Verification items for the finished model (mm, model axes). A direction names the side the tool comes from. Coordinates: 2 decimals unless noted, no trailing zeros. Write each loop counter-clockwise with the first axis right and the second up, starting at its lowest first coordinate (ties: lowest second). Pieces come first, ordered by that corner, then holes. Notation, with made-up numbers: (44, 54) -> (61, 54) arc R26 ccw to (61, 85) -> close; hole circle Ø8 at (40, -20.75). An arc over 180 degrees is marked (long way). Answer in a Markdown table with one row per item.
```python
from build123d import *

# Parameters (mm, degrees)
SKETCH_1_R          = 23.15
EXTRUDE_1_DEPTH     = 1.2
SKETCH_2_R          = 1
CUT_EXTRUDE_1_DEPTH = 1.6


with BuildPart() as part:
    # 草图1 → 凸台-拉伸1 (new body)
    with BuildSketch(Plane(origin=(0, 0, 0), x_dir=(1, 0, 0), z_dir=(0, 1, 0))):
        with Locations(Location((0, 0, 0), (0, 0, 270))):
            Circle(SKETCH_1_R)
    extrude(amount=EXTRUDE_1_DEPTH)

    # 草图2 → 切除-拉伸1 (cut)
    with BuildSketch(Plane(origin=(0, 1.2, 0), x_dir=(1, 0, 0), z_dir=(0, 1, 0))):
        with Locations(Location((0, 20.5, 0), (0, 0, 270))):
            Circle(SKETCH_2_R)
        with Locations(Location((14.495689014, 14.495689014, 0), (0, 0, 270))):
            Circle(SKETCH_2_R)
        with Locations(Location((14.495689014, -14.495689014, 0), (0, 0, 270))):
            Circle(SKETCH_2_R)
        with Locations(Location((0, -20.5, 0), (0, 0, 270))):
            Circle(SKETCH_2_R)
        with Locations(Location((-14.495689014, -14.495689014, 0), (0, 0, 270))):
            Circle(SKETCH_2_R)
        with Locations(Location((-14.495689014, 14.495689014, 0), (0, 0, 270))):
            Circle(SKETCH_2_R)
        Polygon((23.15, 0), (23.15, 4), (9.15, 4), (9.15, -4), (23.15, -4), align=None)
    extrude(amount=-CUT_EXTRUDE_1_DEPTH, mode=Mode.SUBTRACT)


solid = part.part
```
1. Mould release check, pull along Z, two halves, no side actions. Record for faces 3 (the cylindrical face through (-15.472, 0.608, 14.279)), 4 (the cylindrical face through (-23.13, 0.59, -0.96)), 5 (the flat face through (0, 1.2, 0)): released by +Z, released by -Z, zero draft, split by the parting line, or undercut.
Geometry says:
| item | result |
|---|---|
| face 3 | undercut |
| face 4 | split by the parting line |
| face 5 | zero draft |
2. Section check B-B, the plane z = 20.5. Record the boundary of the cut face in (x, y).
Geometry says:
| item | result |
|---|---|
| outline | (-10.76, 0) -> (-1, 0) -> (-1, 1.2) -> (-10.76, 1.2) -> close; (1, 0) -> (10.76, 0) -> (10.76, 1.2) -> (1, 1.2) -> close |
3. Section check A-A, the plane x = 0. Record the boundary of the cut face in (y, z).
Geometry says:
| item | result |
|---|---|
| outline | (0, -23.15) -> (1.2, -23.15) -> (1.2, -21.5) -> (0, -21.5) -> close; (0, -19.5) -> (1.2, -19.5) -> (1.2, 19.5) -> (0, 19.5) -> close; (0, 21.5) -> (1.2, 21.5) -> (1.2, 23.15) -> (0, 23.15) -> close |
4. Tool access check on faces 1 (the cylindrical face through (15.487, 0.608, 14.366)), 2 (the flat face through (16, 1, 4)). Record the directions out of +Z, -Z, +X, -X, +Y, -Y that give a thin tool (end or side, any length) a straight path to the whole face; none if there is none.
Geometry says:
| item | result |
|---|---|
| face 1 | +Y, -Y |
| face 2 | +X, +Y, -Y |
5. Thickness scan on line 1 (Z direction, x = 12, y = 0.85); line 2 (Z direction, x = -0.5, y = 0.15); line 3 (Z direction, x = 11, y = 0.35). Record the ranges inside material, lowest first. Write a range as from..to.
Geometry says:
| item | result |
|---|---|
| line 1 | -19.8..-4, 4..19.8 |
| line 2 | -23.14..-21.37, -19.63..19.63, 21.37..23.14 |
| line 3 | -20.37..-4, 4..20.37 |
6. Section check D-D, the plane x = 19. Record the boundary of the cut face in (y, z), plus the area to 3 significant figures.
Geometry says:
| item | result |
|---|---|
| outline | (0, -13.23) -> (1.2, -13.23) -> (1.2, -4) -> (0, -4) -> close; (0, 4) -> (1.2, 4) -> (1.2, 13.23) -> (0, 13.23) -> close |
| area | 22.1 mm^2 |
7. Section check C-C, the plane y = 0.85. Record the boundary of the cut face in (x, z), plus the area to 3 significant figures.
Geometry says:
| item | result |
|---|---|
| outline | (9.15, -4) -> (9.15, 4) -> (22.8, 4) arc R23.15 ccw (long way) to (22.8, -4) -> close; hole circle Ø2 at (-14.5, -14.5); hole circle Ø2 at (-14.5, 14.5); hole circle Ø2 at (0, -20.5); hole circle Ø2 at (0, 20.5); hole circle Ø2 at (14.5, -14.5); hole circle Ø2 at (14.5, 14.5) |
| area | 1,550 mm^2 |
8. Depth check by flat-ended pin: P1, Ø3, axis at x = 0, z = -20.5, coming from the +Y side; P2, Ø0.6, axis at x = 14, y = 0.5, coming from the +Z side; P3, Ø0.6, axis at y = 1, z = 0.5, coming from the +X side. Enter the tip coordinate at first touch or a pass-through.
Geometry says:
| item | result |
|---|---|
| P1 | y = 1.2 |
| P2 | z = 18.66 |
| P3 | x = 9.15 |
